Design review of the part built by this model. Coordinates are the model's own, in mm. Face numbers are marked on the shaded views. A direction names the side the tool comes from. Give positions to 0.01 mm unless a question says otherwise; leave off trailing zeros. Loops run counter-clockwise (first coordinate to the right, second up) from the corner with the lowest first, then second, coordinate; pieces in that order, holes last. Notation, with made-up numbers: (64.5, -26.75) - (111.5, -26.75) arc R10 cw to (111.5, -21.75) - close; hole circle Ø7 at (52.5, 59). An arc over 180 degrees is marked (long way). Write each question's results on one line, items separated by ' | '.
```python
from build123d import *

# Parameters (mm, degrees)
EXTRUDE_1_DEPTH     = 6
SKETCH_2_R          = 1.6
CUT_EXTRUDE_1_DEPTH = 22


with BuildPart() as part:
    # Эскиз1 → Бобышка-Вытянуть1 (new body)
    with BuildSketch(Plane(origin=(0, 0, 0), x_dir=(1, 0, 0), z_dir=(0, 1, 0))):
        Polygon((-9.65, 9), (-9.65, 12), (11.35, 12), (11.35, 9), (19.5, 9), (19.5, -9), (11.35, -9), (11.35, -12), (-9.65, -12), (-9.65, -9), (-20.5, -9), (-20.5, 9), align=None)
        with BuildLine():
            Line((6.406364979, -4.542135759), (-7.593635021, -4.542135759))
            ThreePointArc((-7.593635021, -4.542135759), (-9.714955364, -3.663456103), (-10.593635021, -1.542135759))
            Line((-10.593635021, -1.542135759), (-10.593635021, 1.457864241))
            ThreePointArc((-10.593635021, 1.457864241), (-9.714955364, 3.579184584), (-7.593635021, 4.457864241))
            Line((-7.593635021, 4.457864241), (6.406364979, 4.457864241))
            ThreePointArc((6.406364979, 4.457864241), (8.527685323, 3.579184584), (9.406364979, 1.457864241))
            Line((9.406364979, 1.457864241), (9.406364979, -1.542135759))
            ThreePointArc((9.406364979, -1.542135759), (8.527685323, -3.663456103), (6.406364979, -4.542135759))
        make_face(mode=Mode.SUBTRACT)
        with BuildLine():
            Line((4.5, 6.4), (-5.5, 6.4))
            ThreePointArc((-5.5, 6.4), (-6.560660172, 6.839339828), (-7, 7.9))
            Line((-7, 7.9), (-7, 8.1))
            ThreePointArc((-7, 8.1), (-6.560660172, 9.160660172), (-5.5, 9.6))
            Line((-5.5, 9.6), (4.5, 9.6))
            ThreePointArc((4.5, 9.6), (5.560660172, 9.160660172), (6, 8.1))
            Line((6, 8.1), (6, 7.9))
            ThreePointArc((6, 7.9), (5.560660172, 6.839339828), (4.5, 6.4))
        make_face(mode=Mode.SUBTRACT)
        with BuildLine():
            Line((4.5, -9.6), (-5.5, -9.6))
            ThreePointArc((-5.5, -9.6), (-6.560660172, -9.160660172), (-7, -8.1))
            Line((-7, -8.1), (-7, -7.9))
            ThreePointArc((-7, -7.9), (-6.560660172, -6.839339828), (-5.5, -6.4))
            Line((-5.5, -6.4), (4.5, -6.4))
            ThreePointArc((4.5, -6.4), (5.560660172, -6.839339828), (6, -7.9))
            Line((6, -7.9), (6, -8.1))
            ThreePointArc((6, -8.1), (5.560660172, -9.160660172), (4.5, -9.6))
        make_face(mode=Mode.SUBTRACT)
    extrude(amount=EXTRUDE_1_DEPTH)

    # Эскиз2 → Вырез-Вытянуть1 (cut, through all)
    with BuildSketch(Plane(origin=(0, 0, -9), x_dir=(-1, 0, 0), z_dir=(0, 0, -1))):
        with Locations((-15.35, 3)):
            Circle(SKETCH_2_R)
        with Locations((16.65, 3)):
            Circle(SKETCH_2_R)
    extrude(amount=-CUT_EXTRUDE_1_DEPTH, mode=Mode.SUBTRACT)


solid = part.part
```
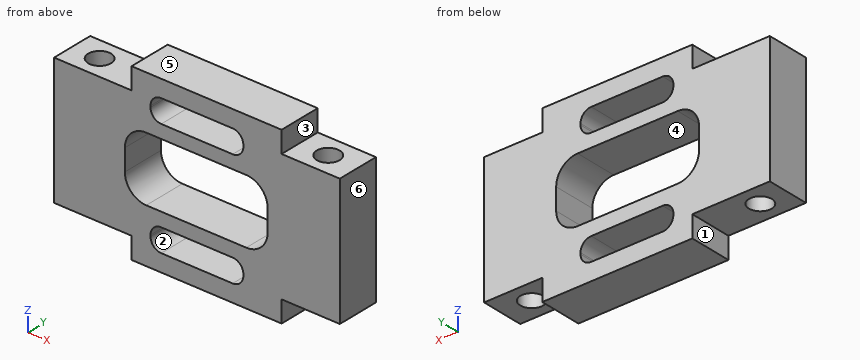
Item 1: We need section D-D on y = 3. Give the number of separate pieces and of enclosed holes in the cut face, then the cut area to 3 significant figures.
Output values:
separate pieces: 3 | enclosed holes: 3 | area: 479 mm²
Item 2: Tool access review of the marked faces 1, 2 and 3: name each direction out of +Z, -Z, +X, -X, +Y, -Y from which nothing blocks a thin tool from reaching the whole face with its end or side.
Output values:
face 1: -Z, -X, +Y, -Y | face 2: +Y, -Y | face 3: +Z, +X, +Y, -Y
Item 3: Clearance check with flat-ended pins moving along their axes: P1, Ø3.5, axis at y = 3, z = 10.5, coming from the +X side; P2, Ø3, axis at x = -16.5, y = 2.5, coming from the -Z side; P3, Ø3, axis at x = 17.5, y = 2, coming from the +Z side. State where each tip first meets the part, or that it passes through.
Output values:
P1: stops at x = 19.5 | P2: stops at z = -9 | P3: stops at z = 9
Item 4: Wall thickness on probe 1 along Z at (x, y) = (-1, 3.85); probe 2 along Y at (x, z) = (15.35, 0.25); probe 3 along X at (y, z) = (2.5, 1.75): over which ranges is each line inside the solid? List them lowest first.
Output values:
probe 1: z = -12 to -9.6, -6.4 to -4.46, 4.54 to 6.4, 9.6 to 12 | probe 2: y = 0 to 1.4, 4.6 to 6 | probe 3: x = -20.5 to -18.17, -15.13 to -10.59, 9.4 to 13.83, 16.87 to 19.5
Item 5: We need section B-B on z = 6. Give the boundary of the cut face in (x, y).
Output values:
outline: (-20.5, 0) - (19.5, 0) - (19.5, 6) - (-20.5, 6) - close; hole circle Ø3.2 at (-16.65, 3); hole circle Ø3.2 at (15.35, 3)
Item 6: We need section C-C on x = 15.35. Give the boundary of the cut face in (y, z), then the cut area to 3 significant figures.
Output values:
outline: (0, -9) - (1.4, -9) - (1.4, 9) - (0, 9) - close; (4.6, -9) - (6, -9) - (6, 9) - (4.6, 9) - close | area: 50.4 mm²
Item 7: We need section A-A on x = 2.5. Give the boundary of the cut face in (y, z), then the cut area to 3 significant figures.
Output values:
outline: (0, -12) - (6, -12) - (6, -9.6) - (0, -9.6) - close; (0, -6.4) - (6, -6.4) - (6, -4.46) - (0, -4.46) - close; (0, 4.54) - (6, 4.54) - (6, 6.4) - (0, 6.4) - close; (0, 9.6) - (6, 9.6) - (6, 12) - (0, 12) - close | area: 51.6 mm²
Item 8: Draft analysis for pull direction X (two halves, no side actions). For the marked faces 4, 5 and 6, state which applies: +X half, -X half, draft (parallel to the pull), parting line (faces both ways), or undercut.
Output values:
face 4: undercut | face 5: draft | face 6: +X half
